Source: CAD feature listing. Evaluate the final solid. Frame: model axes, mm. A direction names the side the tool comes from. Round coordinates to 2 decimals unless told otherwise and drop trailing zeros. Order: outer loops, then holes, each group sorted by start corner. A loop starts at its lowest first (then second) coordinate and runs counter-clockwise, first axis right, second up. Notation, with made-up numbers: M 13.5,88.25 L 56.5,88.25 A21 cw 56.5,112.25 Z; hole C -20.5,-26.5 d8. An arc over 180 degrees is marked long. Answer in a Markdown table with one row per item. Add a question column.
```python
from build123d import *

# Parameters (mm, degrees)
ESQUISSE1_W                      = 140
ESQUISSE1_H                      = 40
BOSS_EXTRU_1_DEPTH               = 3
BOSS_EXTRU_5_DEPTH               = 10
CHANFREIN1_SIZE                  = 6
ESQUISSE15_R                     = 2
ENL_V_MAT_EXTRU_7_DEPTH          = 81.703159789
ESQUISSE18_W                     = 60
ESQUISSE18_H                     = 2
BOSS_EXTRU_6_DEPTH               = 4
CONG_2_R                         = 5
CONG_3_R                         = 2
SYM_TRIE1_OUTLINE_W              = 4
SYM_TRIE1_OUTLINE_H              = 2
SYM_TRIE1_DEPTH                  = 62.191181732
SYM_TRIE1_START                  = 68
SYM_TRIE1_2_DEPTH                = 2
SYM_TRIE1_START_2                = 66.191181932
SYM_TRIE1_3_OUTLINE_W            = 10
SYM_TRIE1_3_OUTLINE_H            = 2
SYM_TRIE1_3_OUTLINE_W_2          = 4
SYM_TRIE1_3_DEPTH                = 1.808818068
SYM_TRIE1_START_3                = 62
SYM_TRIE1_4_OUTLINE_W            = 4
SYM_TRIE1_4_OUTLINE_H            = 2
SYM_TRIE1_4_DEPTH                = 6
SYM_TRIE1_5_OUTLINE_W            = 6
SYM_TRIE1_5_OUTLINE_H            = 2
SYM_TRIE1_5_DEPTH                = 0.191181732
SYM_TRIE1_START_4                = -20
SYM_TRIE1_6_DEPTH                = 2
SYM_TRIE1_START_5                = 2
SYM_TRIE1_7_DEPTH                = 5
CONG_4_R                         = 5
ESQUISSE2_W                      = 19
ESQUISSE2_H                      = 10
BOSS_EXTRU_7_DEPTH               = 20
ESQUISSE19_W                     = 15
ESQUISSE19_H                     = 6
ENL_V_MAT_EXTRU_8_DEPTH          = 77.347887987
CONG_5_R                         = 1
R_P_TITION_LIN_AIRE1_COUNT       = 3
R_P_TITION_LIN_AIRE1_PITCH       = 50
CONG_5_OF_R_P_TITION_LIN_AIRE1_R = 1
ESQUISSE23_R                     = 4.5
BOSS_EXTRU_9_DEPTH               = 20
ESQUISSE24_R                     = 2.70848906
ESQUISSE24_R_2                   = 2.902672956
ENL_V_MAT_EXTRU_10_DEPTH         = 77.347887987


with BuildPart() as part:
    # Esquisse1 → Boss.-Extru.1 (new body)
    with BuildSketch(Plane(origin=(0, 0, 0), x_dir=(1, 0, 0), z_dir=(0, 1, 0))):
        Rectangle(ESQUISSE1_W, ESQUISSE1_H)
    extrude(amount=BOSS_EXTRU_1_DEPTH)

    # Esquisse13 → Boss.-Extru.5 (add)
    with BuildSketch(Plane(origin=(0, 3, 0), x_dir=(1, 0, 0), z_dir=(0, 1, 0))):
        Polygon((-70, 20), (-60, 20), (-60, 18), (-68, 18), (-68, 10), (-70, 10), align=None)
    extrude(amount=BOSS_EXTRU_5_DEPTH)

    # Chanfrein1
    chanfrein1_edges = [part.edges().sort_by_distance(p)[0] for p in [
        (-69, 13, -10),
    ]]
    chamfer(chanfrein1_edges, length=CHANFREIN1_SIZE)

    # Esquisse15 → Enlèv. mat.-Extru.7 (cut, through all)
    with BuildSketch(Plane.XY.offset(-18)):
        with Locations((-64.191181832, 8)):
            Circle(ESQUISSE15_R)
    extrude(amount=-ENL_V_MAT_EXTRU_7_DEPTH, mode=Mode.SUBTRACT)

    # Esquisse18 → Boss.-Extru.6 (add)
    with BuildSketch(Plane(origin=(0, 3, 0), x_dir=(1, 0, 0), z_dir=(0, 1, 0))):
        Polygon((-68, 10), (-68, -18), (0, -18), (0, -20), (-70, -20), (-70, 10), align=None)
        with Locations((-30, 19)):
            Rectangle(ESQUISSE18_W, ESQUISSE18_H)
    extrude(amount=BOSS_EXTRU_6_DEPTH)

    # Congé2
    cong_2_edges = [part.edges().sort_by_distance(p)[0] for p in [
        (-68, 5, 18),
        (-70, 3.5, 20),
    ]]
    fillet(cong_2_edges, radius=CONG_2_R)

    # Congé3
    cong_3_edges = [part.edges().sort_by_distance(p)[0] for p in [
        (-60, 13, -19),
        (-69, 13, -16),
        (-69, 7, -10),
        (-60, 7, -19),
    ]]
    fillet(cong_3_edges, radius=CONG_3_R)

    # Symétrie1: read off the stored shape, not the designer's step
    # Symétrie1 outline → Symétrie1 (add)
    with BuildSketch(Plane.YZ):
        with Locations((5, -19)):
            Rectangle(SYM_TRIE1_OUTLINE_W, SYM_TRIE1_OUTLINE_H)
        with Locations((5, 19)):
            Rectangle(SYM_TRIE1_OUTLINE_W, SYM_TRIE1_OUTLINE_H)
    extrude(amount=SYM_TRIE1_DEPTH)

    # Sym_trie1 2 outline → Sym_trie1 2 (add)
    with BuildSketch(Plane.YZ.offset(SYM_TRIE1_START)):
        with BuildLine():
            Line((13, -20), (13, -16.828427125))
            ThreePointArc((13, -16.828427125), (12.847759065, -16.06306026), (12.414213562, -15.414213562))
            Line((12.414213562, -15.414213562), (7.585786438, -10.585786438))
            ThreePointArc((7.585786438, -10.585786438), (7.152240935, -9.93693974), (7, -9.171572875))
            Line((7, -9.171572875), (7, 20))
            Line((7, 20), (3, 20))
            Line((3, 20), (3, -20))
            Line((3, -20), (13, -20))
        make_face()
    extrude(amount=SYM_TRIE1_2_DEPTH)

    # Sym_trie1 3 outline → Sym_trie1 3 (add)
    with BuildSketch(Plane.YZ.offset(SYM_TRIE1_START_2)):
        with Locations((8, -19)):
            Rectangle(SYM_TRIE1_3_OUTLINE_W, SYM_TRIE1_3_OUTLINE_H)
        with Locations((5, 19)):
            Rectangle(SYM_TRIE1_3_OUTLINE_W_2, SYM_TRIE1_3_OUTLINE_H)
    extrude(amount=SYM_TRIE1_3_DEPTH)

    # Sym_trie1 4 outline → Sym_trie1 4 (add)
    with BuildSketch(Plane.YZ.offset(SYM_TRIE1_START_3)):
        with Locations((5, 19)):
            Rectangle(SYM_TRIE1_4_OUTLINE_W, SYM_TRIE1_4_OUTLINE_H)
    extrude(amount=SYM_TRIE1_4_DEPTH)

    # Sym_trie1 5 outline → Sym_trie1 5 (add)
    with BuildSketch(Plane.YZ.offset(SYM_TRIE1_START_3)):
        with Locations((10, -19)):
            Rectangle(SYM_TRIE1_5_OUTLINE_W, SYM_TRIE1_5_OUTLINE_H)
    extrude(amount=SYM_TRIE1_5_DEPTH)

    # Sym_trie1 6 outline → Sym_trie1 6 (add)
    with BuildSketch(Plane.XY.offset(SYM_TRIE1_START_4)):
        with BuildLine():
            ThreePointArc((62, 13), (60.585786438, 12.414213562), (60, 11))
            Line((60, 11), (60, 9))
            ThreePointArc((60, 9), (59.414213562, 7.585786438), (58, 7))
            Line((58, 7), (62, 7))
            Line((62, 7), (62, 13))
        make_face()
        with BuildLine():
            Line((66.191181932, 13), (62.191181732, 13))
            Line((62.191181732, 13), (62.191181832, 8))
            ThreePointArc((62.191181832, 8), (64.191181832, 10), (66.191181832, 8))
            Line((66.191181832, 8), (66.191181932, 13))
        make_face()
        with BuildLine():
            Line((62.191181832, 8), (62.191181732, 3))
            Line((62.191181732, 3), (66.191181932, 3))
            Line((66.191181932, 3), (66.191181832, 8))
            ThreePointArc((66.191181832, 8), (64.191181832, 6), (62.191181832, 8))
        make_face()
    extrude(amount=SYM_TRIE1_6_DEPTH)

    # Sym_trie1 7 outline → Sym_trie1 7 (add)
    with BuildSketch(Plane(origin=(0, 0, 0), x_dir=(1, 0, 0), z_dir=(0, 1, 0)).offset(SYM_TRIE1_START_5)):
        with BuildLine():
            Line((68, -18), (68, -13))
            ThreePointArc((68, -13), (66.535533906, -16.535533906), (63, -18))
            Line((63, -18), (68, -18))
        make_face()
    extrude(amount=SYM_TRIE1_7_DEPTH)

    # Congé4
    cong_4_edges = [part.edges().sort_by_distance(p)[0] for p in [
        (70, 3.5, 20),
    ]]
    fillet(cong_4_edges, radius=CONG_4_R)

    # Esquisse2 → Boss.-Extru.7 (add)
    with BuildSketch(Plane(origin=(0, 3, 0), x_dir=(1, 0, 0), z_dir=(0, 1, 0))):
        with Locations((-50, 5)):
            Rectangle(ESQUISSE2_W, ESQUISSE2_H)
    boss_extru_7 = extrude(amount=BOSS_EXTRU_7_DEPTH)

    # Esquisse19 → Enlèv. mat.-Extru.8 (cut, through all)
    with BuildSketch(Plane(origin=(0, 23, 0), x_dir=(1, 0, 0), z_dir=(0, 1, 0))):
        with Locations((-50, 5)):
            Rectangle(ESQUISSE19_W, ESQUISSE19_H)
    enl_v_mat_extru_8 = extrude(amount=-ENL_V_MAT_EXTRU_8_DEPTH, mode=Mode.SUBTRACT)

    # Congé5
    cong_5_edges = [part.edges().sort_by_distance(p)[0] for p in [
        (-40.5, 13, 0),
        (-40.5, 13, -10),
        (-59.5, 13, -10),
        (-59.5, 13, 0),
    ]]
    fillet(cong_5_edges, radius=CONG_5_R)

    # Répétition linéaire1: Boss.-Extru.7, Enlèv. mat.-Extru.8 ×3
    with Locations(*[(i * R_P_TITION_LIN_AIRE1_PITCH, 0, 0) for i in range(1, R_P_TITION_LIN_AIRE1_COUNT)]):
        add(boss_extru_7)
        add(enl_v_mat_extru_8, mode=Mode.SUBTRACT)

    # Congé5 of Répétition linéaire1
    cong_5_of_r_p_tition_lin_aire1_edges = [part.edges().sort_by_distance(p)[0] for p in [
        (9.5, 13, 0),
        (9.5, 13, -10),
        (-9.5, 13, -10),
        (-9.5, 13, 0),
        (59.5, 13, 0),
        (59.5, 13, -10),
        (40.5, 13, -10),
        (40.5, 13, 0),
    ]]
    fillet(cong_5_of_r_p_tition_lin_aire1_edges, radius=CONG_5_OF_R_P_TITION_LIN_AIRE1_R)

    # Esquisse23 → Boss.-Extru.9 (add)
    with BuildSketch(Plane(origin=(0, 3, 0), x_dir=(1, 0, 0), z_dir=(0, 1, 0))):
        with Locations(Location((-24.856422556, -10, 0), (0, 0, 270))):
            Circle(ESQUISSE23_R)
        with Locations(Location((28.032520994, -10, 0), (0, 0, 270))):
            Circle(ESQUISSE23_R)
    extrude(amount=BOSS_EXTRU_9_DEPTH)

    # Esquisse24 → Enlèv. mat.-Extru.10 (cut, through all)
    with BuildSketch(Plane(origin=(0, 23, 0), x_dir=(1, 0, 0), z_dir=(0, 1, 0))):
        with Locations(Location((-24.856422556, -10, 0), (0, 0, 270))):
            Circle(ESQUISSE24_R)
        with Locations(Location((28.032520994, -10, 0), (0, 0, 270))):
            Circle(ESQUISSE24_R_2)
    extrude(amount=-ENL_V_MAT_EXTRU_10_DEPTH, mode=Mode.SUBTRACT)


solid = part.part
```
(1) Cut plane A-A (x = 46.5). Return loops of the section in (y, z), and give its area (3 significant figures).
(2) Line query: line 1 (X direction, y = 15.5, z = 10); line 2 (X direction, y = 15.75, z = -7); line 3 (Z direction, x = -25, y = 9.75). Output: solid intervals per line, ascending. Write a range as from..to.
(3) Cut plane B-B (z = 10). Return loops of the section in (x, y).
(4) Pin query (flat end, axial travel): pin 1 (5 mm diameter, centred on y = 11.5, z = -6, fed in from -X); pin 2 (6 mm diameter, centred on x = 36.5, z = -13.5, fed in from +Y); pin 3 (4 mm diameter, centred on x = 40.5, y = 11.5, fed in from +Z). Return the tip coordinate at first contact, or that it passes through.
(5) Cut plane C-C (y = 17.5). Count the separate pieces of the cut face and the enclosed holes in it, and give its area (3 significant figures).
(6) Access query for faces 5 (the face through (-67, 5, 16)), 6 (the face through (0, 12, -8)), 7 (the face through (62.193, 7.912, -19.014)), 8 (the face through (68, 3, 19)), 9 (the face through (-1, 4, 20)). Directions: +Z, -Z, +X, -X, +Y, -Y. A direction counts if a zero-diameter tool reaches every point of the face in a straight line with its end or side. Return the directions, or none.
(7) Draft query along X for faces 1 (the face through (-69, 3, 18)), 2 (the face through (-66, 13, -19)), 3 (the face through (50, 13, -10)), 4 (the face through (-1, 6, -18)). Return one class per face: +X half, -X half, draft (parallel to the pull), parting line (faces both ways), or undercut.
Answer list:
| question | item | result |
|---|---|---|
| 1 | outline | M 0,-20 L 7,-20 L 7,-18 L 3,-18 L 3,-10 L 23,-10 L 23,-8 L 0,-8 Z; M 0,-2 L 23,-2 L 23,0 L 3,0 L 3,18 L 7,18 L 7,20 L 0,20 Z |
| 1 | area | 198 mm² |
| 2 | line 1 | -29.36..-27.56, -22.15..-20.36, 23.53..25.13, 30.94..32.53 |
| 2 | line 2 | -59.5..-57.5, -42.5..-40.5, -9.5..-7.5, 7.5..9.5, 40.5..42.5, 57.5..59.5 |
| 2 | line 3 | 5.5..7.3, 12.7..14.5 |
| 3 | outline | M -70,0 L -27.56,0 L -27.56,23 L -29.36,23 L -29.36,3 L -68,3 L -68,7 L -70,7 Z; M -22.15,0 L 25.13,0 L 25.13,23 L 23.53,23 L 23.53,3 L -20.36,3 L -20.36,23 L -22.15,23 Z; M 30.94,0 L 70,0 L 70,7 L 68,7 L 68,3 L 32.53,3 L 32.53,23 L 30.94,23 Z |
| 4 | pin 1 | x = -59.5 |
| 4 | pin 2 | y = 3 |
| 4 | pin 3 | z = 0 |
| 5 | separate pieces | 5 |
| 5 | enclosed holes | 5 |
| 5 | area | 375 mm² |
| 6 | face 5 | +Y |
| 6 | face 6 | +Y, -Y |
| 6 | face 7 | -Z |
| 6 | face 8 | +Z, +X, +Y, -Y |
| 6 | face 9 | +Z, +X, -X, +Y, -Y |
| 7 | face 1 | -X half |
| 7 | face 2 | draft |
| 7 | face 3 | undercut |
| 7 | face 4 | undercut |
